Read the model definition and answer for the solid it produces. Units are mm, in the model's axes. A direction names the side the tool comes from. Give positions to 0.01 mm unless a question says otherwise; leave off trailing zeros. Loops run counter-clockwise (first coordinate to the right, second up) from the corner with the lowest first, then second, coordinate; pieces in that order, holes last. Notation, with made-up numbers: (27.5, -16) - (73.5, -16) arc R29 ccw to (73.5, 9) - close; hole circle Ø8 at (52, 59). An arc over 180 degrees is marked (long way). Write each question's results on one line, items separated by ' | '. Start each with the question number.
Q1. The part is cut by section B-B, the plane y = -19. Write down the section's boundary in (x, z) (3 decimals), plus the area to 3 significant figures.
Q2. Given pin 1 (12 mm diameter, centred on x = 14, y = -16.5, fed in from +Z), flat-ended and moving along its own axis, determine where the tip first touches the part or whether it passes through.
Q3. The part is cut by section D-D, the plane y = -2. Write down the section's boundary in (x, z) (3 decimals).
Q4. For faces 1 (the flat face through (-38.1, 0, 0)), 2 (the cylindrical face through (3.17, -12.52, 0.14)), 3 (the cylindrical face through (-0.53, 3.03, -0.95)), determine the directions among +Z, -Z, +X, -X, +Y, -Y from which every point of the face is accessible in a straight line to the end or side of a thin tool.
Q5. Find the intervals of material crossed by line 1 (Y direction, x = 23, z = 0) (3 decimals); line 2 (Y direction, x = 7.5, z = -1.25); line 3 (X direction, y = -22, z = 2.5), in increasing order. Write a range as from..to.
Q6. The part is cut by section A-A, the plane z = 0. Write down the section's boundary in (x, y) (3 decimals), plus the area to 3 significant figures.
Autodesk Inventor part; units mm, degrees
ref_plane "Work Plane1" through (0, -31.75, 0) normal (0, -1, 0) x (1, 0, 0)
ref_plane "YZ Plane" through (0, 0, 0) normal (1, 0, 0) x (0, 1, 0)
ref_plane "XZ Plane" through (0, 0, 0) normal (0, 1, 0) x (-1, 0, 0)
sketch "Sketch1" plane through (0, 0, 0) normal (1, 0, 0) x (0, 1, 0)
  circle A0 centre (0, 0) radius 3.175
  dimension "postHoleDiam" = 6.35
extrude "Extrusion1" add sketch "Sketch1" along normal mid plane 76.2
sketch "Sketch3" plane through (0, 0, 0) normal (0, 1, 0) x (-1, 0, 0)
  circle A0 centre (0, 0) radius 3.175
  line L0 (38.1, 3.175) -> (-38.1, 3.175)
extrude "Extrusion2" add sketch "Sketch3" against normal blind 25.4
ref_plane "Work Plane1" through (0, -31.75, 0) normal (0, -1, 0) x (1, 0, 0)
sketch "Sketch5" plane through (0, 0, 0) normal (0, 0, 1) x (1, 0, 0)
  line L0 (-3.175, -25.4) -> (3.175, -25.4)
  arc A0 (-3.175, -25.4) -> (0, -28.575) centre (0, -25.4) ccw
  line L1 (0, -25.4) -> (0, -28.575)
  line L2 (-3.175, -25.4) -> (0, -25.4)
  point P0 (0, 0)
revolve "Revolution1" add sketch "Sketch5" angle 360 about axis through (0, -25.4, 0) along (0, -1, 0)
equation "\"postHoleDiam\" = hopperHoleDiam"
equation "\"camDiam\" = 6.35"
equation "\"hopperHoleDiam\" = 6.35"
properties part number "camPost"
Check sheet entries:
1) outline: circle Ø6.35 at (0, 0) | area: 31.7 mm^2
2) pin 1: passes through
3) outline: (-38.1, -2.466) - (-2, -2.466) arc R3.175 ccw to (2, -2.466) - (38.1, -2.466) - (38.1, 2.466) - (2, 2.466) arc R3.175 ccw to (-2, 2.466) - (-38.1, 2.466) - close
4) face 1: +Z, -Z, -X, +Y, -Y | face 2: -Y | face 3: none
5) line 1: y = -3.175..3.175 | line 2: y = -2.92..2.92 | line 3: x = -1.96..1.96
6) outline: (-38.1, -3.175) - (-3.175, -3.175) - (-3.175, -25.4) arc R3.175 ccw to (3.175, -25.4) - (3.175, -3.175) - (38.1, -3.175) - (38.1, 3.175) - (-38.1, 3.175) - close | area: 641 mm^2
